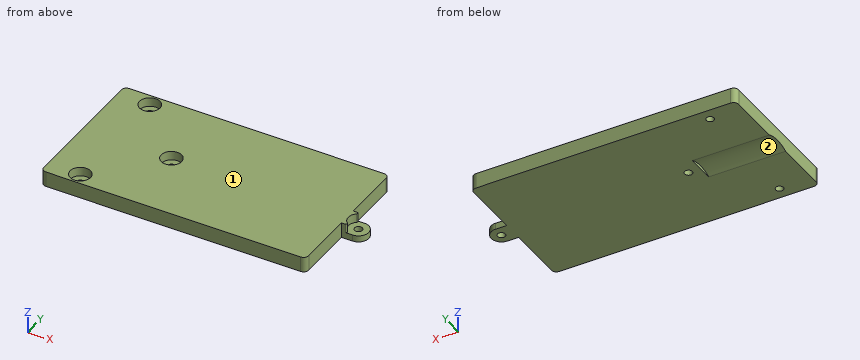
```python
from build123d import *

# Parameters (mm, degrees)
BOSS_EXTRUDE1_DEPTH      = 1.5
BOSS_EXTRUDE1_DEPTH_BACK = 1.5
SKETCH1_R                = 2.000000000000003
SKETCH2_R                = 0.7500000000000021
SKETCH2_R_2              = 0.7500000000000003
SKETCH2_R_3              = 0.750000000000002
CUT_EXTRUDE1_DEPTH       = 9.500000000000002
SKETCH3_R                = 1.9999999999999996
SKETCH3_R_2              = 0.7500000000000021
SKETCH3_R_3              = 2.0000000000000004
SKETCH3_R_4              = 0.7500000000000003
SKETCH3_R_5              = 2.000000000000003
SKETCH3_R_6              = 0.750000000000002
CUT_EXTRUDE2_DEPTH       = 1.75
FILLET1_R                = 0.25
CUT_EXTRUDE5_DEPTH       = 6.999999999999993
CUT_EXTRUDE6_DEPTH       = 15.000000000000004
FILLET2_R                = 1


with BuildPart() as part:
    # Sketch1 → Boss-Extrude1 (new, two sides: drawn at the far end of the back side and taken through both)
    with BuildSketch(Plane.XY.offset(-BOSS_EXTRUDE1_DEPTH_BACK)):
        Polygon((-26.000000000000007, -14.235000000000003), (-26.000000000000007, 14.234999999999996), (25.999999999999993, 14.235000000000003), (25.999999999999993, -14.234999999999996), align=None)
        with Locations((27.999999999999993, 1.1e-16)):
            Circle(SKETCH1_R)
        with BuildLine():
            Line((25.999999999999993, 1.8438584e-09), (25.999999999999993, -2))
            Line((25.999999999999993, -2), (27.99999999999995, -2))
            ThreePointArc((27.99999999999995, -2.000000000000003), (26.585786436974978, -1.4142135617211795), (25.99999999999999, 1.84385875e-09))
        make_face()
        with BuildLine():
            Line((25.999999999999993, 2), (25.999999999999993, 1.8438584e-09))
            ThreePointArc((25.99999999999999, 1.84385875e-09), (26.585786438278785, 1.414213563024986), (27.999999999999954, 2.000000000000003))
            Line((27.999999999999954, 2), (25.999999999999993, 2))
        make_face()
    extrude(amount=BOSS_EXTRUDE1_DEPTH + BOSS_EXTRUDE1_DEPTH_BACK)

    # Sketch2 → Cut-Extrude1 (cut)
    with BuildSketch(Plane.XY.offset(1.5)):
        with Locations((-19.500000000000007, 11.735000000000005)):
            Circle(SKETCH2_R)
        with Locations((-8.500000000000004, 0)):
            Circle(SKETCH2_R_2)
        with Locations((-19.500000000000007, -11.734999999999996)):
            Circle(SKETCH2_R)
        with Locations((27.999999999999993, -4.3e-16)):
            Circle(SKETCH2_R_3)
    extrude(amount=-CUT_EXTRUDE1_DEPTH, mode=Mode.SUBTRACT)

    # Sketch3 → Cut-Extrude2 (cut)
    # profile 1 of 4: a face of its own
    with BuildSketch(Plane.XY.offset(1.5)):
        with Locations((-19.500000000000007, 11.735000000000005)):
            Circle(SKETCH3_R)
        with Locations((-19.500000000000007, 11.735000000000005)):
            Circle(SKETCH3_R_2, mode=Mode.SUBTRACT)
    # profile 2 of 4: a face of its own
    with BuildSketch(Plane.XY.offset(1.5)):
        with Locations((-8.500000000000004, 0)):
            Circle(SKETCH3_R_3)
        with Locations((-8.500000000000004, 0)):
            Circle(SKETCH3_R_4, mode=Mode.SUBTRACT)
    # profile 3 of 4: a face of its own
    with BuildSketch(Plane.XY.offset(1.5)):
        with Locations((-19.500000000000007, -11.734999999999996)):
            Circle(SKETCH3_R)
        with Locations((-19.500000000000007, -11.734999999999996)):
            Circle(SKETCH3_R_2, mode=Mode.SUBTRACT)
    # profile 4 of 4: a face of its own
    with BuildSketch(Plane.XY.offset(1.5)):
        with Locations((27.999999999999993, -4.3e-16)):
            Circle(SKETCH3_R_5)
        with Locations((27.999999999999993, -4.3e-16)):
            Circle(SKETCH3_R_6, mode=Mode.SUBTRACT)
    extrude(amount=-CUT_EXTRUDE2_DEPTH, mode=Mode.SUBTRACT)

    # Fillet1
    fillet1_edges = [part.edges().sort_by_distance(p)[0] for p in [
        (27.999999999999915, 2.0000000000000018, 0.625),
        (27.99999999999991, -2.000000000000002, 0.625),
    ]]
    fillet(fillet1_edges, radius=FILLET1_R)

    # Sketch7 → Cut-Extrude5 (cut)
    with BuildSketch(Plane.XY.offset(1.5)):
        Polygon((25.999999999999993, -14.234999999999996), (25.999999999999993, -2), (25.84999999999999, -2), (25.84999999999999, -14.084999999999996), (-25.85, -14.084999999999999), (-25.850000000000005, 14.084999999999994), (25.84999999999999, 14.085000000000003), (25.84999999999999, 2), (25.999999999999993, 2), (25.999999999999993, 14.235000000000003), (-26.000000000000007, 14.234999999999996), (-26.000000000000007, -14.235000000000003), align=None)
    extrude(amount=-CUT_EXTRUDE5_DEPTH, mode=Mode.SUBTRACT)

    # Sketch8 → Cut-Extrude6 (cut)
    with BuildSketch(Plane.ZY.offset(25.850000000000005)):
        with BuildLine():
            Line((-1.4999999999999996, 2.749545416973646), (-1.4999999999999996, 0))
            Line((-1.5, 3.5e-16), (-0.8999999999999995, 2.1e-16))
            ThreePointArc((-0.8999999999999995, 1.73e-15), (-1.0517444219386114, 1.4071247279470998), (-1.5000000000000586, 2.749545416973634))
        make_face()
        with BuildLine():
            Line((-1.4999999999999996, -2.749545416973639), (-1.4999999999999996, 0))
            Line((-1.4999999999999996, 0), (-1.4999999999999996, 2.749545416973646))
            ThreePointArc((-1.5000000000000586, 2.749545416973634), (-14.100000000000001, 2.54e-15), (-1.5000000000000577, -2.7495454169736293))
        make_face()
        with BuildLine():
            Line((-0.8999999999999995, 2.1e-16), (-1.5, 3.5e-16))
            Line((-1.4999999999999996, 0), (-1.4999999999999996, -2.749545416973639))
            ThreePointArc((-1.5000000000000577, -2.7495454169736293), (-1.0517444219386123, -1.4071247279470989), (-0.8999999999999995, 1.2e-16))
        make_face()
    extrude(amount=-CUT_EXTRUDE6_DEPTH, mode=Mode.SUBTRACT)

    # Fillet2
    fillet2_edges = [part.edges().sort_by_distance(p)[0] for p in [
        (25.849999999999987, -14.084999999999996, 0),
        (25.84999999999999, 14.085000000000003, 0),
        (-25.850000000000005, 14.084999999999994, 0),
        (-25.85, -14.085, 0),
    ]]
    fillet(fillet2_edges, radius=FILLET2_R)


solid = part.part
```
Geometry: final body of the model. Coordinates: model frame, mm. Face numbers are marked on the shaded views. Round coordinates to 2 decimals unless told otherwise and drop trailing zeros. Order: outer loops, then holes, each group sorted by start corner. A loop starts at its lowest first (then second) coordinate and runs counter-clockwise, first axis right, second up. Notation, with made-up numbers: (-31, 62) -> (23, 62) arc R12 ccw to (23, 78) -> close; hole circle Ø10 at (63.25, 69.25). An arc over 180 degrees is marked (long way). Use CSV: the item, a comma, the result in double quotes. Start each with the question number.
1) Section C-C (x = -8.5). Return the cut outline in (y, z) (3 decimals).
2) Section B-B (x = -19.5). Return the cut outline in (y, z) (3 decimals), and give its area (3 significant figures).
3) Section A-A (y = 0). Return the cut outline in (x, z), and give its area (3 significant figures).
4) First-contact query: pin 1 Ø1.7 at (x, y) = (28, 0) entering from +Z; pin 2 Ø4.5 at (x, y) = (-19.5, -11.735) entering from +Z; pin 3 Ø0.6 at (x, z) = (26.5, 0.5) entering from -Y; pin 4 Ø0.9 at (y, z) = (7.5, 0) entering from +X. Flat tips, straight axial feed; report the tip coordinate or a pass-through.
5) Section D-D (z = 1). Return the cut outline in (x, y) (3 decimals), and give its area (3 significant figures).
6) Material intervals for line 1 along Y through (x, z) = (-19.5, -0.7) (3 decimals); line 2 along Y through (x, z) = (28, -0.75); line 3 along Y through (x, z) = (-7, 1.2) (3 decimals), sorted ascending. Write a range as from..to.
7) Draft query along Y for the marked faces 1 and 2. Return one class per face: +Y half, -Y half, draft (parallel to the pull), parting line (faces both ways), or undercut.
Returned:
1,outline,"(-14.085, -1.5) -> (-0.75, -1.5) -> (-0.75, -0.25) -> (-2, -0.25) -> (-2, 1.5) -> (-14.085, 1.5) -> close; (0.75, -1.5) -> (14.085, -1.5) -> (14.085, 1.5) -> (2, 1.5) -> (2, -0.25) -> (0.75, -0.25) -> close"
2,outline,"(-14.085, -1.5) -> (-12.485, -1.5) -> (-12.485, -0.25) -> (-13.735, -0.25) -> (-13.735, 1.5) -> (-14.085, 1.5) -> close; (-10.985, -1.5) -> (-2.75, -1.5) arc R6.6 cw to (2.75, -1.5) -> (10.985, -1.5) -> (10.985, -0.25) -> (9.735, -0.25) -> (9.735, 1.5) -> (-9.735, 1.5) -> (-9.735, -0.25) -> (-10.985, -0.25) -> close; (12.485, -1.5) -> (14.085, -1.5) -> (14.085, 1.5) -> (13.735, 1.5) -> (13.735, -0.25) -> (12.485, -0.25) -> close"
2,area,"64.5 mm²"
3,outline,"(-25.85, -0.9) -> (-10.85, -0.9) -> (-10.85, -1.5) -> (-9.25, -1.5) -> (-9.25, -0.25) -> (-10.5, -0.25) -> (-10.5, 1.5) -> (-25.85, 1.5) -> close; (-7.75, -1.5) -> (27.25, -1.5) -> (27.25, -0.25) -> (26, -0.25) -> (26, 1.5) -> (-6.5, 1.5) -> (-6.5, -0.25) -> (-7.75, -0.25) -> close; (28.75, -1.5) -> (30, -1.5) -> (30, -0.25) -> (28.75, -0.25) -> close"
3,area,"141 mm²"
4,pin 1,"stops at z = -0.25"
4,pin 2,"stops at z = 1.5"
4,pin 3,"stops at y = -2"
4,pin 4,"stops at x = 25.85"
5,outline,"(-25.85, -13.085) arc R1 ccw to (-24.85, -14.085) -> (24.85, -14.085) arc R1 ccw to (25.85, -13.085) -> (25.85, -2) -> (26.586, -2) arc R0.25 ccw to (26.743, -1.556) arc R2 cw to (26.743, 1.556) arc R0.25 ccw to (26.586, 2) -> (25.85, 2) -> (25.85, 13.085) arc R1 ccw to (24.85, 14.085) -> (-24.85, 14.085) arc R1 ccw to (-25.85, 13.085) -> close; hole circle Ø4 at (-19.5, -11.735); hole circle Ø4 at (-19.5, 11.735); hole circle Ø4 at (-8.5, 0)"
5,area,"1,420 mm²"
6,line 1,"y = -14.085..-12.485, -10.985..10.985, 12.485..14.085"
6,line 2,"y = -2..-0.75, 0.75..2"
6,line 3,"y = -14.085..-1.323, 1.323..14.085"
7,face 1,"draft"
7,face 2,"undercut"
